Design review of the part built by this model. Coordinates are the model's own, in mm. Coordinates: 2 decimals unless noted, no trailing zeros. Write each loop counter-clockwise with the first axis right and the second up, starting at its lowest first coordinate (ties: lowest second). Pieces come first, ordered by that corner, then holes.
Q1. For pin 1 Ø2 at (y, z) = (23.5, 7.5) entering from -X; pin 2 Ø1.5 at (x, y) = (26, 8.5) entering from +Z; pin 3 Ø3 at (y, z) = (25, 3.5) entering from -X, all flat-tipped, find the tip position at first contact; note any pin that passes through.
Q2. Take a section at C-C, the plane x = 33. Write out the cut boundary in (y, z), plus the area to 3 significant figures.
Q3. Take a section at A-A, the plane y = 28. Write out the cut boundary in (x, z).
Q4. For L1, parallel to X at y = 15.5, z = 4; L2, parallel to X at y = 17.5, z = 3; L3, parallel to Z at x = 34, y = 4, list the stretches that pass through material, from the lowest coordinate up.
Q5. Take a section at B-B, the plane z = 2.5. Write out the cut boundary in (x, y), plus the area to 3 significant figures.
from build123d import *

# Parameters (mm, degrees)
F0_W     = 34.9964526249
F0_H     = 47.8031225502
F1_DEPTH = 24.638
F3_DEPTH = 25.4
F4_DEPTH = 89.408
F5_R     = 5.08
F6_R     = 5.08


with BuildPart() as f1:
    # F0 (on Top) → F1 (new body)
    with BuildSketch(Plane.XY):
        with Locations((18.5126164579, 23.9015612751)):
            Rectangle(F0_W, F0_H)
    extrude(amount=F1_DEPTH)

    # F2 (on face) → F3 (join)
    with BuildSketch(Plane(origin=(0, 47.8031225502, 0), x_dir=(-1, 0, 0), z_dir=(0, 1, 0))):
        Polygon((-36.0108427703, 24.638), (-36.0108427703, 0), (-30.9388898313, 5.7059428655), (-23.4577655792, 9.0027097613), (-15.7230421901, 9.0027097613), (-9.6367038786, 6.21313788), (-4.437955562, 0), (-1.0143901454, 0), (-1.0143901454, 24.638), align=None)
    extrude(amount=F3_DEPTH)

    # F4 (cut): a face of the model
    f4_faces = [f1.faces().sort_by_distance(p)[0] for p in [
        (18.0448789955, 73.2031225502, 14.9299983871),
    ]]
    extrude(f4_faces, amount=-F4_DEPTH, mode=Mode.SUBTRACT)

    # F5
    f5_edges = [f1.edges().sort_by_distance(p)[0] for p in [
        (23.457766, 23.901561, 9.00271),
    ]]
    fillet(f5_edges, radius=F5_R)

    # F6
    f6_edges = [f1.edges().sort_by_distance(p)[0] for p in [
        (15.723042, 23.901561, 9.00271),
        (9.636704, 23.901561, 6.213138),
        (30.93889, 23.901561, 5.705943),
    ]]
    fillet(f6_edges, radius=F6_R)


solid = f1.part
Responses:
1. pin 1: stops at x = 10.3
1. pin 2: stops at z = 8.21
1. pin 3: stops at x = 6.11
2. outline: (0, 0) - (47.8, 0) - (47.8, 3.39) - (0, 3.39) - close
2. area: 162 mm2
3. outline: (4.44, 0) - (36.01, 0) - (31.67, 4.88) arc R5.08 ccw to (29.93, 6.15) - (24.44, 8.57) arc R5.08 ccw to (22.39, 9) - (16.83, 9) arc R5.08 ccw to (14.72, 8.54) - (10.68, 6.69) arc R5.08 ccw to (8.9, 5.33) - close
4. L1: x = 7.78 to 32.46
4. L2: x = 6.95 to 33.34
4. L3: z = 0 to 2.26
5. outline: (6.53, 0) - (33.79, 0) - (33.79, 47.8) - (6.53, 47.8) - close
5. area: 1,300 mm2
